CAD build for the part. Positions are in the model's coordinates, mm. A direction names the side the tool comes from. Give positions to 0.01 mm unless a question says otherwise; leave off trailing zeros. Loops run counter-clockwise (first coordinate to the right, second up) from the corner with the lowest first, then second, coordinate; pieces in that order, holes last.
Item 1: Saw through at C-C on z = 16.5. Give the cut face in (x, y).
Item 2: Drop flat-ended pins along their axis: P1, Ø1.5, axis at x = 0, z = 6.5, coming from the -Y side; P2, Ø1.5, axis at x = 1, z = 7, coming from the +Y side; P3, Ø10, axis at x = -8.5, z = 13.5, coming from the +Y side. Give the stop position or say it passes through.
Item 3: Which spindle directions (+Z, -Z, +X, -X, +Y, -Y) get a long thin tool onto all of the face, cutting with end or side? Do faces 1 (the flat face through (24, -8, 25.4)), 2 (the flat face through (0, 2.5, 7)). Say none if no direction does.
Item 4: Probe probe 1 along Y at (x, z) = (0, 15.5); probe 2 along Z at (x, y) = (-21.5, 4); probe 3 along Y at (x, z) = (-16, 7.5). List the from-to ranges inside material, lowest first.
Item 5: Saw through at D-D on z = 2.5. Give the cut face in (x, y), plus the area to 3 significant figures.
Item 6: Saw through at A-A on x = 0. Give the cut face in (y, z), plus the area to 3 significant figures.
Item 7: Mould opens along X. For faces 3 (the cylindrical face through (-5.85, -26.36, 15.06)), 4 (the cylindrical face through (23.846, 7.509, 15.54)), 5 (the flat face through (0, 0, 0)), 6 (the flat face through (-2.5, 0, 7)) say: released by +X, released by -X, zero draft, split by the parting line, or undercut.
from build123d import *

# Parameters (mm, degrees)
F0_R     = 27
F5_DEPTH = 25.4
F1_R     = 25
F2_DEPTH = 20
F3_R     = 5
F4_W     = 5
F4_H     = 5
F6_DEPTH = 3


with BuildPart() as f5:
    # F0 (on Top) → F5 (new body)
    with BuildSketch(Plane.XY):
        Circle(F0_R)
    extrude(amount=F5_DEPTH)

    # F1 (on face) → F2 (cut)
    with BuildSketch(Plane.XY.offset(25.4)):
        Circle(F1_R)
    extrude(amount=-F2_DEPTH, mode=Mode.SUBTRACT)

    # F3
    f3_edges = [f5.edges().sort_by_distance(p)[0] for p in [
        (-27, 0, 0),
    ]]
    fillet(f3_edges, radius=F3_R)

    # F4 (on face) → F6 (join)
    with BuildSketch(Plane.XY.offset(5.4)):
        Rectangle(F4_W, F4_H)
    extrude(amount=F6_DEPTH)


solid = f5.part
Results below:
1. outline: circle Ø54 at (0, 0); hole circle Ø50 at (0, 0)
2. P1: stops at y = -27
2. P2: stops at y = 27
2. P3: stops at y = 26.77
3. face 1: +Z, +X, -X, +Y, -Y
3. face 2: +Z
4. probe 1: y = -27 to -25, 25 to 27
4. probe 2: z = 0 to 5.4
4. probe 3: y = -21.75 to -19.21, 19.21 to 21.75
5. outline: circle Ø52.66 at (0, 0)
5. area: 2,180 mm2
6. outline: (-27, 5) arc R5 ccw to (-22, 0) - (22, 0) arc R5 ccw to (27, 5) - (27, 25.4) - (25, 25.4) - (25, 5.4) - (2.5, 5.4) - (2.5, 8.4) - (-2.5, 8.4) - (-2.5, 5.4) - (-25, 5.4) - (-25, 25.4) - (-27, 25.4) - close
6. area: 376 mm2
7. face 3: split by the parting line
7. face 4: undercut
7. face 5: zero draft
7. face 6: undercut
